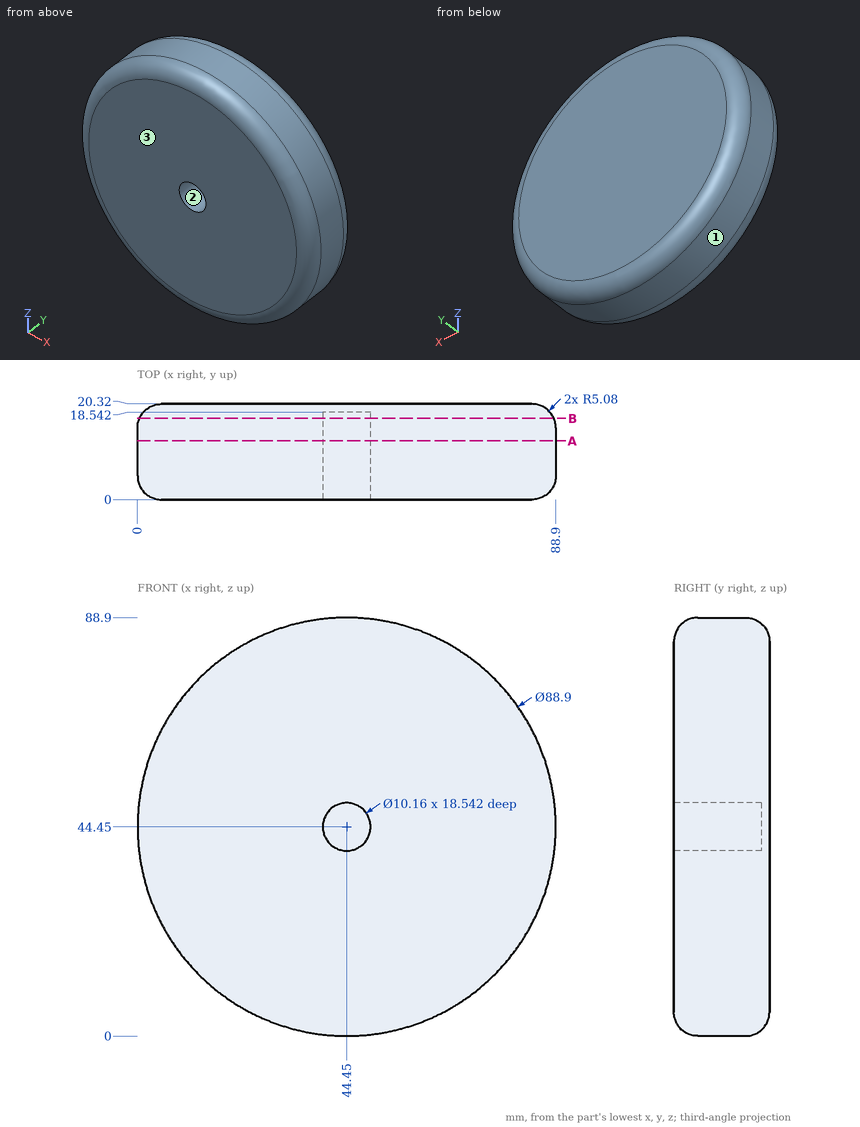
Design review of the part shown in the three views and the two pictorial views. Dimensions are in mm from the part's minimum x, y and z. Give positions to 0.01 mm unless a question says otherwise; leave off trailing zeros. Write each loop counter-clockwise with the first axis right and the second up, starting at its lowest first coordinate (ties: lowest second). Pieces come first, ordered by that corner, then holes. Notation, with made-up numbers: M 31,50 L 42,50 A25 cw 42,78 Z; hole C 54,-5 d4. An arc over 180 degrees is marked long. Return JSON: item names as keys, results as strings. Group by question number.
Item 1: Clearance check with flat-ended pins moving along their axes: pin 1 Ø10 at (y, z) = (5.5, 78.5) entering from -X; pin 2 Ø12 at (y, z) = (9.5, 54) entering from -X; pin 3 Ø2 at (x, y) = (15.5, 14.5) entering from -Z; pin 4 Ø8 at (x, z) = (46, 46.5) entering from -Y. State where each tip first meets the part, or that it passes through.
Item 2: The part is to be moulded in two halves that separate along Z. For the marked faces 1, 2 and 3, say which applies: pulls with the +Z half, pulls with the -Z half, needs draft (parallel to the pull), parting line crosses it, or undercut.
Item 3: Take a section at A-A (y = 12.5). Give the boundary of the cut face in (x, z).
Item 4: Wall thickness on line 1 along Z through (x, y) = (44.45, 10); line 2 along X through (y, z) = (7.5, 26); line 3 along Z through (x, y) = (54.5, 6): over which ranges is each line inside the solid? List them lowest first.
Item 5: Take a section at B-B (y = 17.25). Give the boundary of the cut face in (x, z).
Return value:
{
 "1": {"pin 1": "stops at x = 10.81", "pin 2": "stops at x = 0.14", "pin 3": "stops at z = 9.89", "pin 4": "stops at y = 0"},
 "2": {"face 1": "parting line crosses it", "face 2": "undercut", "face 3": "needs draft"},
 "3": {"outline": "C 44.45,44.45 d88.9; hole C 44.45,44.45 d10.16"},
 "4": {"line 1": "z = 0 to 39.37, 49.53 to 88.9", "line 2": "x = 4.01 to 84.89", "line 3": "z = 1.15 to 87.75"},
 "5": {"outline": "C 44.45,44.45 d88.07; hole C 44.45,44.45 d10.16"}
}
